Autodesk Inventor part; units mm, degrees
ref_plane "YZ Plane" through (0, 0, 0) normal (1, 0, 0) x (0, 1, 0)
ref_plane "XZ Plane" through (0, 0, 0) normal (0, 1, 0) x (-1, 0, 0)
ref_plane "XY Plane" through (0, 0, 0) normal (0, 0, 1) x (1, 0, 0)
sketch "Sketch1" plane through (0, 0, 0) normal (0, 1, 0) x (-1, 0, 0)
  circle A0 centre (0, 0) radius 65
  dimension "d0" = 130
extrude "Extrusion1" add sketch "Sketch1" along normal blind 7
sketch "Sketch2" plane through (0, 7, 0) normal (0, 1, 0) x (1, 0, 0)
  circle A0 centre (-54, -5.0532) radius 3
  circle A1 centre (-34.6106, -41.7569) radius 3
  circle A2 centre (5.0532, -54) radius 3
  circle A3 centre (41.7569, -34.6106) radius 3
  circle A4 centre (54, 5.0532) radius 3
  circle A5 centre (34.6106, 41.7569) radius 3
  circle A6 centre (-5.0532, 54) radius 3
  circle A7 centre (-41.7569, 34.6106) radius 3
  point P0 (0, 0)
  dimension "d3" = 6
  dimension "d4" = 54
  dimension "d7" = 360
extrude "Extrusion2" cut sketch "Sketch2" against normal through all
sketch "Sketch3" plane through (0, 7, 0) normal (0, 1, 0) x (1, 0, 0)
  circle A0 centre (-51.2366, -17.0532) radius 1.5
  circle A1 centre (-54, -5.0532) radius 3
  circle A2 centre (17.0532, -51.2366) radius 1.5
  circle A3 centre (51.2366, 17.0532) radius 1.5
  circle A4 centre (-17.0532, 51.2366) radius 1.5
  circle A5 centre (-34.6106, -41.7569) radius 3
  point P0 (0, 0)
  dimension "d13" = 3
  dimension "d16" = 360
  dimension "d31" = 12
  dimension "d33" = 54
extrude "Extrusion3" cut sketch "Sketch3" against normal through all contours A0 | A2 | A3 | A4
sketch "Sketch4" plane through (0, 0, 0) normal (0, -1, 0) x (1, 0, 0)
  circle A0 centre (17.0532, 51.2366) radius 3.5
  circle A1 centre (17.0532, 51.2366) radius 1.5
  circle A2 centre (-51.2366, 17.0532) radius 3.5
  circle A3 centre (-17.0532, -51.2366) radius 3.5
  circle A4 centre (51.2366, -17.0532) radius 3.5
  point P0 (0, 0)
  dimension "d20" = 7
  dimension "d23" = 360
extrude "Extrusion4" cut sketch "Sketch4" against normal blind 2
sketch "Sketch5" plane through (0, 7, 0) normal (0, 1, 0) x (1, 0, 0)
  circle A0 centre (0, 0) radius 6
  dimension "d27" = 12
extrude "Extrusion5" add sketch "Sketch5" along normal blind 2
properties part number "bay container 8 bottom"
Check sheet for the modelled part. Datum: model origin and axes. Units: mm. A direction names the side the tool comes from. Give positions to 0.01 mm unless a question says otherwise; leave off trailing zeros. Loops run counter-clockwise (first coordinate to the right, second up) from the corner with the lowest first, then second, coordinate; pieces in that order, holes last. Notation, with made-up numbers: M -25.75,-11.75 L 2.25,-11.75 A6 ccw 2.25,-1.75 Z; hole C 13,-12.5 d5. An arc over 180 degrees is marked long. Use a Markdown table: item, result. Add a question column.
Q1. Tool access check on faces 1 (the cylindrical face through (-6, 8, 0)), 2 (the flat face through (-50.5, 2, 15.5)), 3 (the cylindrical face through (-17.378, 4.535, -49.772)). Record the directions out of +Z, -Z, +X, -X, +Y, -Y that give a thin tool (end or side, any length) a straight path to the whole face; none if there is none.
Q2. Go/stop test with flat-tipped pins: pin 1 (2 mm diameter, centred on x = -19.5, z = 30, fed in from +Y); pin 2 (2 mm diameter, centred on x = -52, z = 18, fed in from -Y); pin 3 (1.5 mm diameter, centred on y = 3.5, z = -51.5, fed in from +X); pin 4 (2.5 mm diameter, centred on x = 17.05, z = 51.24, fed in from +Y). Record where each tip stops, or that it passes through.
Q3. Sectioned sample at D-D, the plane x = -28. Record the cut outline in (y, z), then the cut area to 3 significant figures.
Q4. Sectioned sample at C-C, the plane y = 4.25. Give the number of separate pieces and of enclosed holes in the cut face, then the cut area to 3 significant figures.
Q5. Sectioned sample at B-B, the plane z = 0. Record the cut outline in (x, y), then the cut area to 3 significant figures.
Q6. Scan lines: line 1 along X through (y, z) = (4.75, -52.5); line 2 along Y through (x, z) = (57.5, 0.5); line 3 along X through (y, z) = (1.25, 39.5). Record each from-to range of solid material in increasing order. Write a range as [from, to].
Q7. Sectioned sample at A-A, the plane x = 0. Record the cut outline in (y, z).
Verdict:
| question | item | result |
|---|---|---|
| 1 | face 1 | +Y |
| 1 | face 2 | -Y |
| 1 | face 3 | +Y, -Y |
| 2 | pin 1 | y = 7 |
| 2 | pin 2 | y = 2 |
| 2 | pin 3 | x = 40.61 |
| 2 | pin 4 | through |
| 3 | outline | M 0,-58.66 L 7,-58.66 L 7,58.66 L 0,58.66 Z |
| 3 | area | 821 mm^2 |
| 4 | separate pieces | 1 |
| 4 | enclosed holes | 12 |
| 4 | area | 13,000 mm^2 |
| 5 | outline | M -65,0 L 65,0 L 65,7 L 6,7 L 6,9 L -6,9 L -6,7 L -65,7 Z |
| 5 | area | 934 mm^2 |
| 6 | line 1 | [-38.32, -17.86], [-16.24, -7.65], [-2.46, 38.32] |
| 6 | line 2 | [0, 7] |
| 6 | line 3 | [-51.62, -36.59], [-32.63, 51.62] |
| 7 | outline | M 0,-65 L 7,-65 L 7,-6 L 9,-6 L 9,6 L 7,6 L 7,65 L 0,65 Z |
